from build123d import *

# Parameters (mm, degrees)
SKETCH1_R           = 2.275
BOSS_EXTRUDE4_DEPTH = 3.66
SKETCH8_R           = 12.835
BOSS_EXTRUDE5_DEPTH = 8
SKETCH9_R           = 5.9
BOSS_EXTRUDE6_DEPTH = 11.39
SKETCH10_R          = 4
CUT_EXTRUDE3_DEPTH  = 28.533269421


with BuildPart() as part:
    # Sketch1 → Boss-Extrude4 (new body)
    with BuildSketch(Plane(origin=(0, 0, 0), x_dir=(1, 0, 0), z_dir=(0, 1, 0))):
        with BuildLine():
            Line((-6.648675743, 11.449572519), (-18.733599938, 4.431953109))
            ThreePointArc((-18.733599938, 4.431953109), (-21.285, 0), (-18.733599938, -4.431953109))
            Line((-18.733599938, -4.431953109), (-6.648675743, -11.449572519))
            ThreePointArc((-6.648675743, -11.449572519), (-3.442764866, -12.784559831), (0, -13.24))
            Line((0, -13.24), (0, 13.24))
            ThreePointArc((0, 13.24), (-3.442764866, 12.784559831), (-6.648675743, 11.449572519))
        make_face()
        with Locations(Location((-16.16, 0, 0), (0, 0, 270))):
            Circle(SKETCH1_R, mode=Mode.SUBTRACT)
    boss_extrude4 = extrude(amount=BOSS_EXTRUDE4_DEPTH)

    # Mirror2: Boss-Extrude4 across plane
    add(boss_extrude4.mirror(Plane(origin=(0, 0, 0), x_dir=(0, 0, 1), z_dir=(1, 0, 0))))

    # Sketch8 → Boss-Extrude5 (add)
    with BuildSketch(Plane(origin=(0, 0, 0), x_dir=(1, 0, 0), z_dir=(0, 1, 0))):
        with Locations(Location((0, 0, 0), (0, 0, 270))):
            Circle(SKETCH8_R)
    extrude(amount=BOSS_EXTRUDE5_DEPTH)

    # Sketch9 → Boss-Extrude6 (add)
    with BuildSketch(Plane(origin=(0, 0, 0), x_dir=(1, 0, 0), z_dir=(0, 1, 0))):
        with Locations(Location((0, 0, 0), (0, 0, 270))):
            Circle(SKETCH9_R)
    extrude(amount=BOSS_EXTRUDE6_DEPTH)

    # Sketch10 → Cut-Extrude3 (cut, through all)
    with BuildSketch(Plane(origin=(0, 11.39, 0), x_dir=(1, 0, 0), z_dir=(0, 1, 0))):
        with Locations(Location((0, 0, 0), (0, 0, 270))):
            Circle(SKETCH10_R)
    extrude(amount=-CUT_EXTRUDE3_DEPTH, mode=Mode.SUBTRACT)


solid = part.part
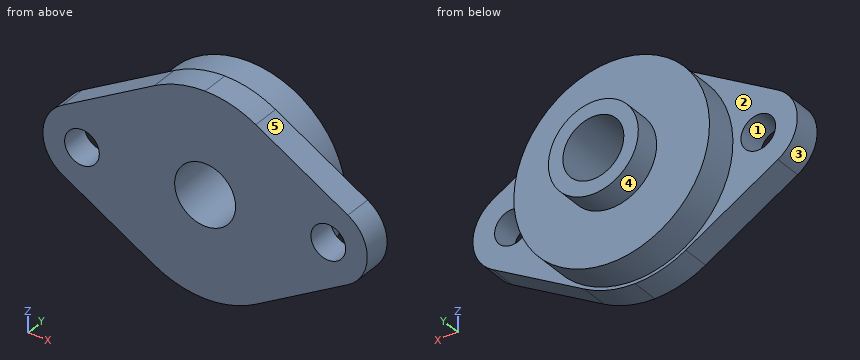
Source: CAD feature listing. Evaluate the final solid. Frame: model axes, mm. Face numbers are marked on the shaded views. A direction names the side the tool comes from. Give positions to 0.01 mm unless a question says otherwise; leave off trailing zeros. Loops run counter-clockwise (first coordinate to the right, second up) from the corner with the lowest first, then second, coordinate; pieces in that order, holes last. Notation, with made-up numbers: (38, -21) -> (56, -21) arc R19 ccw to (56, 5) -> close; hole circle Ø3 at (10.5, 3.25). An arc over 180 degrees is marked (long way). Use a Markdown table: item, result. Add a question column.
1) Line query: line 1 along X through (y, z) = (2.5, -1.25); line 2 along X through (y, z) = (8.5, 0); line 3 along Y through (x, z) = (2.5, 12.25). Output: solid intervals per line, ascending. Write a range as [from, to].
2) Pull-direction query (Z, two-part tool) for the marked faces 1, 2 and 3; classes: +Z half, -Z half, draft (parallel to the pull), parting line (faces both ways), or undercut.
3) Section query D-D, the plane x = 5. Return the cut outline in (y, z), then the cut area to 3 significant figures.
4) Section query B-B, the plane x = 18. Return the cut outline in (y, z).
5) Reachability of the marked faces 4 and 5 from +Z, -Z, +X, -X, +Y, -Y: full face, straight path, thin tool, end or side. Return the list, or none.
6) Section query C-C, the plane y = 10. Return the cut outline in (x, z).
7) First-contact query: pin 1 (6 mm diameter, centred on y = 2, z = -2.5, fed in from +X) (3 decimals); pin 2 (2.5 mm diameter, centred on x = -16.16, z = 0, fed in from -Y). Flat tips, straight axial feed; report the tip coordinate or a pass-through.
8) Section query A-A, the plane z = 0. Return the cut outline in (x, y) (3 decimals), then the cut area to 3 significant figures.
Numbers:
| question | item | result |
|---|---|---|
| 1 | line 1 | x = [-21.13, -18.06], [-14.26, -3.8], [3.8, 14.26], [18.06, 21.13] |
| 1 | line 2 | x = [-5.9, -4], [4, 5.9] |
| 1 | line 3 | y = [0, 8] |
| 2 | face 1 | undercut |
| 2 | face 2 | draft |
| 2 | face 3 | parting line |
| 3 | outline | (0, -12.26) -> (3.66, -12.26) -> (3.66, -11.82) -> (8, -11.82) -> (8, -3.13) -> (11.39, -3.13) -> (11.39, 3.13) -> (8, 3.13) -> (8, 11.82) -> (3.66, 11.82) -> (3.66, 12.26) -> (0, 12.26) -> close |
| 3 | area | 214 mm2 |
| 4 | outline | (0, -4.86) -> (3.66, -4.86) -> (3.66, -1.34) -> (0, -1.34) -> close; (0, 1.34) -> (3.66, 1.34) -> (3.66, 4.86) -> (0, 4.86) -> close |
| 5 | face 4 | +Y |
| 5 | face 5 | +Z, +X, +Y, -Y |
| 6 | outline | circle Ø11.8 at (0, 0); hole circle Ø8 at (0, 0) |
| 7 | pin 1 | stops at x = 21.285 |
| 7 | pin 2 | passes through |
| 8 | outline | (-21.285, 0) -> (-18.435, 0) -> (-18.435, 3.66) -> (-21.285, 3.66) -> close; (-13.885, 0) -> (-4, 0) -> (-4, 11.39) -> (-5.9, 11.39) -> (-5.9, 8) -> (-12.835, 8) -> (-12.835, 3.66) -> (-13.885, 3.66) -> close; (4, 0) -> (13.885, 0) -> (13.885, 3.66) -> (12.835, 3.66) -> (12.835, 8) -> (5.9, 8) -> (5.9, 11.39) -> (4, 11.39) -> close; (18.435, 0) -> (21.285, 0) -> (21.285, 3.66) -> (18.435, 3.66) -> close |
| 8 | area | 183 mm2 |
